```python
from build123d import *

# Parameters (mm, degrees)
F0_W      = 40.5
F0_H      = 40.5
F1_DEPTH  = 1.6
F2_DEPTH  = 22.6
F3_W      = 40.5
F3_H      = 40.5
F4_DEPTH  = 3
F5_W      = 35.6
F5_H      = 14.5
F5_H_2    = 3
F6_DEPTH  = 5
F7_W      = 13.8
F7_H      = 14.5
F7_H_2    = 3
F8_DEPTH  = 5
F9_W      = 4.5
F9_H      = 16
F9_H_2    = 32.5
F10_DEPTH = 5
F11_R     = 1.25
F12_DEPTH = 11


with BuildPart() as f1:
    # F0 (on Top) → F1 (new body)
    with BuildSketch(Plane.XY):
        Rectangle(F0_W, F0_H)
    extrude(amount=F1_DEPTH)

    # F0 (on Top) → F2 (join)
    with BuildSketch(Plane.XY):
        with BuildLine():
            Line((20.5, 22.5), (-20.5, 22.5))
            ThreePointArc((-20.5, 22.5), (-21.9142135624, 21.9142135624), (-22.5, 20.5))
            Line((-22.5, 20.5), (-22.5, -20.5))
            ThreePointArc((-22.5, -20.5), (-21.9142135624, -21.9142135624), (-20.5, -22.5))
            Line((-20.5, -22.5), (20.5, -22.5))
            ThreePointArc((20.5, -22.5), (21.9142135624, -21.9142135624), (22.5, -20.5))
            Line((22.5, -20.5), (22.5, 20.5))
            ThreePointArc((22.5, 20.5), (21.9142135624, 21.9142135624), (20.5, 22.5))
        make_face()
        Rectangle(F0_W, F0_H, mode=Mode.SUBTRACT)
    extrude(amount=F2_DEPTH)

    # F3 (on face) → F4 (join)
    with BuildSketch(Plane.XY.offset(22.6)):
        with BuildLine():
            Line((20.2, 20.85), (-20.2, 20.85))
            ThreePointArc((-20.2, 20.85), (-20.6596194078, 20.6596194078), (-20.85, 20.2))
            Line((-20.85, 20.2), (-20.85, -20.2))
            ThreePointArc((-20.85, -20.2), (-20.6596194078, -20.6596194078), (-20.2, -20.85))
            Line((-20.2, -20.85), (20.2, -20.85))
            ThreePointArc((20.2, -20.85), (20.6596194078, -20.6596194078), (20.85, -20.2))
            Line((20.85, -20.2), (20.85, 20.2))
            ThreePointArc((20.85, 20.2), (20.6596194078, 20.6596194078), (20.2, 20.85))
        make_face()
        Rectangle(F3_W, F3_H, mode=Mode.SUBTRACT)
    extrude(amount=F4_DEPTH)

    # F5 (on face) → F6 (cut)
    with BuildSketch(Plane.YZ.offset(22.5)):
        with Locations((0, 15.35)):
            Rectangle(F5_W, F5_H)
        with Locations((0, 24.1)):
            Rectangle(F5_W, F5_H_2)
    extrude(amount=-F6_DEPTH, mode=Mode.SUBTRACT)

    # F7 (on face) → F8 (cut)
    with BuildSketch(Plane(origin=(-22.5, 0, 0), x_dir=(0, -1, 0), z_dir=(-1, 0, 0))):
        with Locations((0, 15.35)):
            Rectangle(F7_W, F7_H)
        with Locations((0, 24.1)):
            Rectangle(F7_W, F7_H_2)
    extrude(amount=-F8_DEPTH, mode=Mode.SUBTRACT)

    # F9 (on face) → F10 (cut)
    with BuildSketch(Plane.XY.offset(1.6)):
        with Locations((16, 0)):
            Rectangle(F9_W, F9_H)
        with BuildLine():
            Line((20.25, -19.3791561976), (20.25, -17.7208438024))
            ThreePointArc((20.25, -17.7208438024), (17.5, -18.55), (20.25, -19.3791561976))
        make_face()
        with BuildLine():
            ThreePointArc((20.25, -19.3791561976), (20.4361406616, -18.9830127019), (20.5, -18.55))
            ThreePointArc((20.5, -18.55), (20.4361406616, -18.1169872981), (20.25, -17.7208438024))
            Line((20.25, -17.7208438024), (20.25, -19.3791561976))
        make_face()
        with Locations((-16.75, 0)):
            Rectangle(F9_W, F9_H_2)
    extrude(amount=-F10_DEPTH, mode=Mode.SUBTRACT)

    # F11 (on face) → F12 (join)
    with BuildSketch(Plane.XY.offset(1.6)):
        with Locations((16.8683137745, 13.0740953609)):
            Circle(F11_R)
        with Locations((-16.75, 18.4307503104)):
            Circle(F11_R)
        with Locations((-16.75, -18.3533816189)):
            Circle(F11_R)
        with Locations((13.195104897, -16.7595241219)):
            Circle(F11_R)
    extrude(amount=F12_DEPTH)


solid = f1.part
```
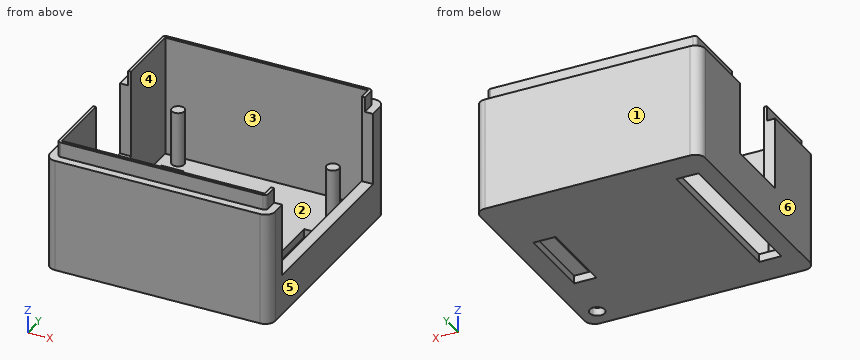
Can you work these out from the model? Positions are in its coordinate system, mm. Face numbers are marked on the shaded views. A direction names the side the tool comes from. Coordinates: 2 decimals unless noted, no trailing zeros. Loops run counter-clockwise (first coordinate to the right, second up) from the corner with the lowest first, then second, coordinate; pieces in that order, holes last.
Item 1: Suppose I cut it at A-A (y = -3). Please give me the cut outline in (x, z), then the cut area to 4 significant figures.
Answers below:
outline: (-22.5, 0) - (-19, 0) - (-19, 1.6) - (-20.25, 1.6) - (-20.25, 8.1) - (-22.5, 8.1) - close; (-14.5, 0) - (13.75, 0) - (13.75, 1.6) - (-14.5, 1.6) - close; (18.25, 0) - (22.5, 0) - (22.5, 8.1) - (20.25, 8.1) - (20.25, 1.6) - (18.25, 1.6) - close
area: 86.85 mm2
Item 2: Suppose I cut it at C-C (x = -16.75). Please give me the cut outline in (y, z).
Answers below:
outline: (-22.5, 0) - (-16.25, 0) - (-16.25, 1.6) - (-17.1, 1.6) - (-17.1, 12.6) - (-19.6, 12.6) - (-19.6, 1.6) - (-20.25, 1.6) - (-20.25, 25.6) - (-20.85, 25.6) - (-20.85, 22.6) - (-22.5, 22.6) - close; (16.25, 0) - (22.5, 0) - (22.5, 22.6) - (20.85, 22.6) - (20.85, 25.6) - (20.25, 25.6) - (20.25, 1.6) - (19.68, 1.6) - (19.68, 12.6) - (17.18, 12.6) - (17.18, 1.6) - (16.25, 1.6) - close
Item 3: Suppose I cut it at B-B (y = -12.5). Please give me the cut outline in (x, z).
Answers below:
outline: (-22.5, 0) - (-19, 0) - (-19, 1.6) - (-20.25, 1.6) - (-20.25, 25.6) - (-20.85, 25.6) - (-20.85, 22.6) - (-22.5, 22.6) - close; (-14.5, 0) - (22.5, 0) - (22.5, 8.1) - (20.25, 8.1) - (20.25, 1.6) - (-14.5, 1.6) - close
Item 4: I'm going to push flat-ended pins straight in: pin 1 (3 mm diameter, centred on y = 5.5, z = 18, fed in from +X); pin 2 (2.5 mm diameter, centred on y = -14.5, z = 24, fed in from -X); pin 3 (2.5 mm diameter, centred on x = 21.5, y = 3.5, fed in from +Z); pin 4 (1.8 mm diameter, centred on x = -21, z = 13.5, fed in from -Y). Where does each tip first touch, or does it pass through?
Answers below:
pin 1: stops at x = -20.25
pin 2: stops at x = -20.85
pin 3: stops at z = 8.1
pin 4: stops at y = -22.5
Item 5: If we mould it in two halves opening along X, with no side actions, what happens to the marked faces 3, 4, 5 and 6? For each: released by +X, released by -X, zero draft, split by the parting line, or undercut.
Answers below:
face 3: undercut
face 4: undercut
face 5: released by +X
face 6: released by -X
Item 6: Suppose I cut it at D-D (z = 3). Please give me the cut outline in (x, y).
Answers below:
outline: (-22.5, -20.5) arc R2 ccw to (-20.5, -22.5) - (20.5, -22.5) arc R2 ccw to (22.5, -20.5) - (22.5, 20.5) arc R2 ccw to (20.5, 22.5) - (-20.5, 22.5) arc R2 ccw to (-22.5, 20.5) - close; circle Ø2.5 at (-16.75, -18.35); circle Ø2.5 at (-16.75, 18.43); circle Ø2.5 at (13.2, -16.76); circle Ø2.5 at (16.87, 13.07); hole (-20.25, -20.25) - (20.25, -20.25) - (20.25, 20.25) - (-20.25, 20.25) - close
Item 7: Which directions (+Z, -Z, +X, -X, +Y, -Y) give clear straight access to the entire face, cutting with the end or side of a thin tool? Please do the marked faces 1 and 2.
Answers below:
face 1: +Z, -Z, +X, -X, +Y
face 2: +Z
Item 8: Please list where these lines run through material, in increasing order: L1, parallel to X at y = -18.5, z = 2; L2, parallel to X at y = -18.55, z = 0.4; L3, parallel to X at y = -11.5, z = 7.25.
Answers below:
L1: x = -22.5 to -20.25, -17.99 to -15.51, 20.25 to 22.5
L2: x = -22.5 to 17.5, 20.5 to 22.5
L3: x = -22.5 to -20.25, 20.25 to 22.5
